Design review of the part shown in the three views and the two pictorial views. Dimensions are in mm from the part's minimum x, y and z. A direction names the side the tool comes from. Coordinates: 2 decimals unless noted, no trailing zeros. Loops run counter-clockwise (first coordinate to the right, second up) from the corner with the lowest first, then second, coordinate; pieces in that order, holes last. Notation, with made-up numbers: (60, -6) -> (103, -6) arc R12 ccw to (103, 2) -> close; hole circle Ø11 at (-20, 33). An arc over 180 degrees is marked (long way). Answer in a Markdown table with one row per item.
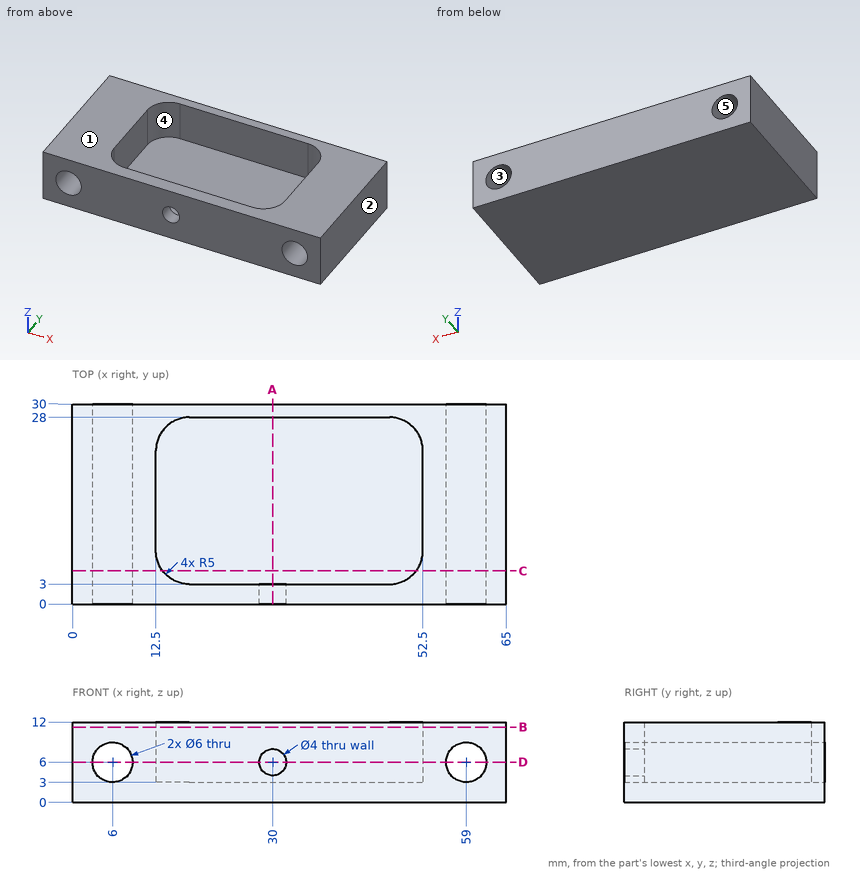
(1) Take a section at A-A on x = 30. Give the boundary of the cut face in (y, z).
Evaluation:
| item | result |
|---|---|
| outline | (0, 0) -> (30, 0) -> (30, 12) -> (28, 12) -> (28, 3) -> (3, 3) -> (3, 4) -> (0, 4) -> close; (0, 8) -> (3, 8) -> (3, 12) -> (0, 12) -> close |
(2) Tool access review of the marked faces 4 and 5: name each direction out of +Z, -Z, +X, -X, +Y, -Y from which nothing blocks a thin tool from reaching the whole face with its end or side.
Evaluation:
| item | result |
|---|---|
| face 4 | +Z |
| face 5 | +Y, -Y |
(3) Take a section at C-C on y = 5. Give the boundary of the cut face in (x, z).
Evaluation:
| item | result |
|---|---|
| outline | (0, 0) -> (65, 0) -> (65, 12) -> (51.5, 12) -> (51.5, 3) -> (13.5, 3) -> (13.5, 12) -> (0, 12) -> close; hole circle Ø6 at (6, 6); hole circle Ø6 at (59, 6) |
(4) To check wall thickness, follow probe 1 along X at (y, z) = (20, 5.75); probe 2 along X at (y, z) = (8, 11); probe 3 along Z at (x, y) = (59, 14). State the ranges of each line that lie inside material, in increasing order.
Evaluation:
| item | result |
|---|---|
| probe 1 | x = 0 to 3.01, 8.99 to 12.5, 52.5 to 56.01, 61.99 to 65 |
| probe 2 | x = 0 to 12.5, 52.5 to 65 |
| probe 3 | z = 0 to 3, 9 to 12 |
(5) Draft analysis for pull direction X (two halves, no side actions). For the marked faces 1, 2 and 3, state which applies: pulls with the +X half, pulls with the -X half, needs draft (parallel to the pull), parting line crosses it, or undercut.
Evaluation:
| item | result |
|---|---|
| face 1 | needs draft |
| face 2 | pulls with the +X half |
| face 3 | undercut |
(6) For pin 1 (1 mm diameter, centred on y = 13.5, z = 9, fed in from -X); pin 2 (1.5 mm diameter, centred on x = 21.5, y = 18, fed in from +Z); pin 3 (5 mm diameter, centred on x = 59, z = 6, fed in from -Y), all flat-tipped, find the tip position at first contact; note any pin that passes through.
Evaluation:
| item | result |
|---|---|
| pin 1 | stops at x = 0 |
| pin 2 | stops at z = 3 |
| pin 3 | passes through |
(7) Take a section at B-B on z = 11.25. Give the boundary of the cut face in (x, y), and give its area (3 significant figures).
Evaluation:
| item | result |
|---|---|
| outline | (0, 0) -> (65, 0) -> (65, 30) -> (0, 30) -> close; hole (12.5, 8) arc R5 ccw to (17.5, 3) -> (47.5, 3) arc R5 ccw to (52.5, 8) -> (52.5, 23) arc R5 ccw to (47.5, 28) -> (17.5, 28) arc R5 ccw to (12.5, 23) -> close |
| area | 971 mm² |
(8) Take a section at D-D on z = 6. Give the boundary of the cut face in (x, y), and give its area (3 significant figures).
Evaluation:
| item | result |
|---|---|
| outline | (0, 0) -> (3, 0) -> (3, 30) -> (0, 30) -> close; (9, 0) -> (28, 0) -> (28, 3) -> (17.5, 3) arc R5 cw to (12.5, 8) -> (12.5, 23) arc R5 cw to (17.5, 28) -> (47.5, 28) arc R5 cw to (52.5, 23) -> (52.5, 8) arc R5 cw to (47.5, 3) -> (32, 3) -> (32, 0) -> (56, 0) -> (56, 30) -> (9, 30) -> close; (62, 0) -> (65, 0) -> (65, 30) -> (62, 30) -> close |
| area | 599 mm² |
